Check sheet for the modelled part. Datum: model origin and axes. Units: mm. A direction names the side the tool comes from. Round coordinates to 2 decimals unless told otherwise and drop trailing zeros. Order: outer loops, then holes, each group sorted by start corner. A loop starts at its lowest first (then second) coordinate and runs counter-clockwise, first axis right, second up.
from build123d import *

# Parameters (mm, degrees)
SKETCH1_R               = 20
BOSS_EXTRUDE1_DEPTH     = 55
SKETCH3_R               = 9
BOSS_EXTRUDE2_DEPTH     = 9
CUT_EXTRUDE1_DEPTH      = 100
CUT_EXTRUDE1_DEPTH_BACK = 2
SKETCH2_R               = 3.5
SKETCH6_R               = 3.5
BOSS_EXTRUDE3_DEPTH     = 28
SKETCH7_R               = 17
CUT_EXTRUDE2_DEPTH      = 3
FILLET2_R               = 2
SKETCH8_R               = 1.5
CUT_EXTRUDE3_DEPTH      = 5


with BuildPart() as part:
    # Sketch1 → Boss-Extrude1 (new body)
    with BuildSketch(Plane.XY):
        Circle(SKETCH1_R)
    extrude(amount=BOSS_EXTRUDE1_DEPTH)

    # Sketch3 → Boss-Extrude2 (add)
    with BuildSketch(Plane.XY.offset(55)):
        Circle(SKETCH3_R)
    extrude(amount=BOSS_EXTRUDE2_DEPTH)

    # Sketch2 → Cut-Extrude1 (cut, two sides: drawn at the far end of the back side and taken through both)
    with BuildSketch(Plane.XY.offset(55).offset(-CUT_EXTRUDE1_DEPTH_BACK)):
        Circle(SKETCH2_R)
    extrude(amount=CUT_EXTRUDE1_DEPTH + CUT_EXTRUDE1_DEPTH_BACK, mode=Mode.SUBTRACT)

    # Sketch6 → Boss-Extrude3 (add)
    with BuildSketch(Plane.XY.offset(53)):
        with Locations(Location((0, 0, 0), (0, 0, 180))):
            Circle(SKETCH6_R)
    extrude(amount=BOSS_EXTRUDE3_DEPTH)

    # Sketch7 → Cut-Extrude2 (cut)
    with BuildSketch(Plane(origin=(0, 0, 0), x_dir=(-1, 0, 0), z_dir=(0, 0, -1))):
        Circle(SKETCH7_R)
    extrude(amount=-CUT_EXTRUDE2_DEPTH, mode=Mode.SUBTRACT)

    # Fillet2
    fillet2_edges = [part.edges().sort_by_distance(p)[0] for p in [
        (-20, 0, 55),
    ]]
    fillet(fillet2_edges, radius=FILLET2_R)

    # Sketch8 → Cut-Extrude3 (cut)
    with BuildSketch(Plane.XY.offset(55)):
        with Locations((0, 13.856406461)):
            Circle(SKETCH8_R)
        with Locations((-12, -6.92820323)):
            Circle(SKETCH8_R)
        with Locations((12, -6.92820323)):
            Circle(SKETCH8_R)
    extrude(amount=-CUT_EXTRUDE3_DEPTH, mode=Mode.SUBTRACT)


solid = part.part
1) Gauge pin test, flat ends, axial feed: pin 1 (3 mm diameter, centred on x = -9.5, y = 4, fed in from -Z); pin 2 (1.5 mm diameter, centred on x = -0.5, y = 13.5, fed in from +Z); pin 3 (10 mm diameter, centred on x = 3.5, y = 15, fed in from -Z); pin 4 (3.5 mm diameter, centred on x = 0, y = 13.86, fed in from +Z). Record the tip position at first contact, or that the pin passes through.
2) Draft check along Y on faces 1 (the face through (0, -4, 64)), 2 (the face through (0, 0, 3)), 3 (the face through (-4.336, -19.524, 26.129)), 4 (the face through (11.67, -8.39, 52.54)). Enter one of: pulls with the +Y half, pulls with the -Y half, needs draft (parallel to the pull), parting line crosses it, or undercut.
3) Sectioned sample at B-B on z = 59.5. Record the cut outline in (x, y), and give its area (3 significant figures).
4) Scan lines: line 1 (Y direction, x = 0, z = 53); line 2 (Z direction, x = 12.5, y = 8); line 3 (Z direction, x = 0, y = -7). Record each from-to range of solid material in increasing order.
5) Sectioned sample at C-C on z = 29.5. Record the cut outline in (x, y), and give its area (3 significant figures).
6) Set-up check for faces 5 (the face through (-3.233, 1.341, 72.381)), 6 (the face through (-9.139, 14.334, 1.479)), 7 (the face through (-9, -15, 0)): record each of +Z, -Z, +X, -X, +Y, -Y from which the full face is reachable in a straight line by a thin tool's end or side.
7) Sectioned sample at A-A on y = 0. Record the cut outline in (x, z), and give its area (3 significant figures).
Values found:
1. pin 1: stops at z = 3
1. pin 2: stops at z = 50
1. pin 3: stops at z = 0
1. pin 4: stops at z = 55
2. face 1: needs draft
2. face 2: undercut
2. face 3: parting line crosses it
2. face 4: undercut
3. outline: circle Ø18 at (0, 0)
3. area: 254 mm2
4. line 1: y = -20 to 12.36, 15.36 to 20
4. line 2: z = 3 to 55
4. line 3: z = 3 to 64
5. outline: circle Ø40 at (0, 0)
5. area: 1,260 mm2
6. face 5: +Z
6. face 6: -Z
6. face 7: -Z, +X, -X, +Y, -Y
7. outline: (-20, 0) - (-17, 0) - (-17, 3) - (17, 3) - (17, 0) - (20, 0) - (20, 53) arc R2 ccw to (18, 55) - (9, 55) - (9, 64) - (3.5, 64) - (3.5, 81) - (-3.5, 81) - (-3.5, 64) - (-9, 64) - (-9, 55) - (-18, 55) arc R2 ccw to (-20, 53) - close
7. area: 2,380 mm2
